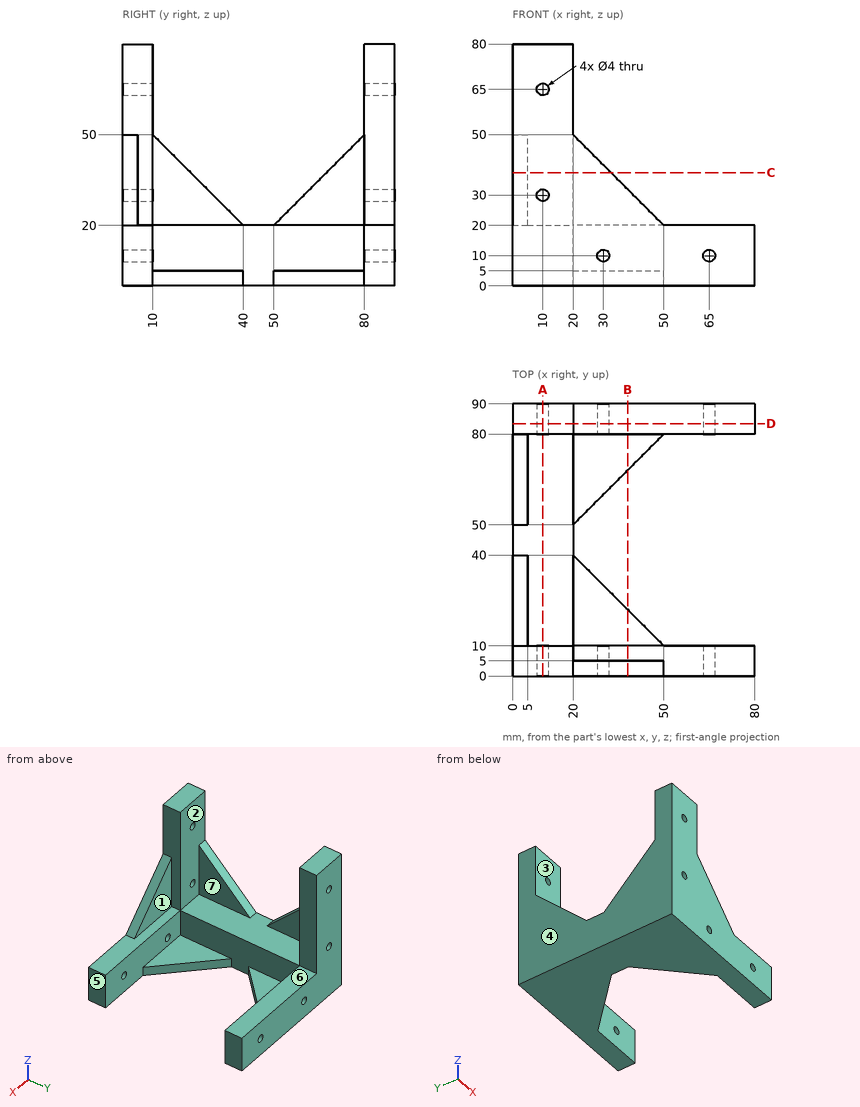
Input: dimensioned drawing with shaded views. Units: mm. Origin: part minimum x, y, z. A direction names the side the tool comes from. Coordinates: 2 decimals unless noted, no trailing zeros. Order: outer loops, then holes, each group sorted by start corner. A loop starts at its lowest first (then second) coordinate and runs counter-clockwise, first axis right, second up.
Item 1: Material intervals for line 1 along Z through (x, y) = (10, 85); line 2 along Y through (x, z) = (10.5, 71.5); line 3 along Z through (x, y) = (30, 84.5), sorted ascending.
Answer:
line 1: z = 0 to 28, 32 to 63, 67 to 80
line 2: y = 0 to 10, 80 to 90
line 3: z = 0 to 8, 12 to 20
Item 2: Section query D-D (y = 83.5). Output: boundary loops of the cut face in (x, z).
Answer:
outline: (0, 0) - (80, 0) - (80, 20) - (20, 20) - (20, 80) - (0, 80) - close; hole circle Ø4 at (10, 30); hole circle Ø4 at (10, 65); hole circle Ø4 at (30, 10); hole circle Ø4 at (65, 10)
Item 3: Access query for the marked faces 5, 6 and 7. Directions: +Z, -Z, +X, -X, +Y, -Y. A direction counts if a zero-diameter tool reaches every point of the face in a straight line with its end or side. Return the directions, or none.
Answer:
face 5: +Z, -Z, +X, +Y, -Y
face 6: +Z, +X, +Y
face 7: +Z, +X
Item 4: Section query B-B (x = 38). Output: boundary loops of the cut face in (y, z).
Answer:
outline: (0, 0) - (22, 0) - (22, 5) - (10, 5) - (10, 20) - (5, 20) - (5, 32) - (0, 32) - close; (68, 0) - (90, 0) - (90, 20) - (80, 20) - (80, 5) - (68, 5) - close
Item 5: Draft query along Y for the marked faces 1, 2, 3 and 4. Return one class per face: released by +Y, released by -Y, zero draft, split by the parting line, or undercut.
Answer:
face 1: released by +Y
face 2: undercut
face 3: undercut
face 4: zero draft
Item 6: Section query C-C (z = 37.5). Output: boundary loops of the cut face in (x, y).
Answer:
outline: (0, 0) - (32.5, 0) - (32.5, 5) - (20, 5) - (20, 10) - (5, 10) - (5, 22.5) - (0, 22.5) - close; (0, 67.5) - (5, 67.5) - (5, 80) - (20, 80) - (20, 90) - (0, 90) - close
Item 7: Section query A-A (x = 10). Output: boundary loops of the cut face in (y, z), then the cut area to 3 significant figures.
Answer:
outline: (0, 0) - (90, 0) - (90, 28) - (80, 28) - (80, 20) - (10, 20) - (10, 28) - (0, 28) - close; (0, 32) - (10, 32) - (10, 63) - (0, 63) - close; (0, 67) - (10, 67) - (10, 80) - (0, 80) - close; (80, 32) - (90, 32) - (90, 63) - (80, 63) - close; (80, 67) - (90, 67) - (90, 80) - (80, 80) - close
area: 2,840 mm2
Item 8: Contact query for flat-ended pins moving along their axis: P1, Ø4, axis at y = 39, z = 10, coming from the +X side; P2, Ø15, axis at x = 39.5, y = 68.5, coming from the +Z side; P3, Ø5, axis at x = 42, y = 85, coming from the +Z side. Output: stop coordinate, or through.
Answer:
P1: stops at x = 20
P2: stops at z = 5
P3: stops at z = 20
